Geometry: final body of the model. Coordinates: model frame, mm. A direction names the side the tool comes from. Round coordinates to 2 decimals unless told otherwise and drop trailing zeros. Write each loop counter-clockwise with the first axis right and the second up, starting at its lowest first coordinate (ties: lowest second). Pieces come first, ordered by that corner, then holes.
from build123d import *

# Parameters (mm, degrees)
F0_W          = 70
F0_H          = 60
F1_DEPTH      = 5
F2_R          = 4
F3_DEPTH      = 3
F4_R          = 1.5
F5_DEPTH      = 3.001
F5_DEPTH_BACK = 5
F6_DEPTH      = 3
F7_DEPTH      = 3
F9_DEPTH      = 5
F11_DEPTH     = 3
F13_DEPTH     = 2.5


with BuildPart() as f1:
    # F0 (on Top) → F1 (new body)
    with BuildSketch(Plane.XY):
        Rectangle(F0_W, F0_H)
    extrude(amount=F1_DEPTH)

    # F2 (on face) → F3 (join)
    with BuildSketch(Plane.XY.offset(5)):
        with Locations((-23.7, 23.1)):
            Circle(F2_R)
        with Locations((-25, -25.1)):
            Circle(F2_R)
        with Locations((27.1, 7.9)):
            Circle(F2_R)
        with Locations((27.1, -20)):
            Circle(F2_R)
    extrude(amount=F3_DEPTH)

    # F4 (on face) → F5 (cut, two sides)
    with BuildSketch(Plane.XY.offset(5)) as f5_sk:
        with Locations((-23.7, 23.1)):
            Circle(F4_R)
        with Locations((27.1, 7.9)):
            Circle(F4_R)
        with Locations((27.1, -20)):
            Circle(F4_R)
        with Locations((-25, -25.1)):
            Circle(F4_R)
    extrude(amount=F5_DEPTH, mode=Mode.SUBTRACT)
    extrude(f5_sk.sketch, amount=-F5_DEPTH_BACK, mode=Mode.SUBTRACT)

    # F6 (add): a face of the model
    f6_faces = [f1.faces().sort_by_distance(p)[0] for p in [
        (0, -30, 2.5),
    ]]
    extrude(f6_faces, amount=F6_DEPTH)

    # F7 (add): a face of the model
    f7_faces = [f1.faces().sort_by_distance(p)[0] for p in [
        (0, 30, 2.5),
    ]]
    extrude(f7_faces, amount=F7_DEPTH)

    # F8 (on face) → F9 (cut)
    with BuildSketch(Plane.XY.offset(5)):
        with BuildLine():
            Line((-14.3054683646, -1.7219720702), (-14.0948043176, -1.5533969252))
            ThreePointArc((-14.0948043176, -1.5533969252), (-14.2033899748, -1.6336185148), (-14.3054683646, -1.7219720702))
        make_face()
        with BuildLine():
            Line((0.0942490372, 9.8008030979), (-14.0948043176, -1.5533969252))
            Line((-14.0948043176, -1.5533969252), (-14.3054683646, -1.7219720702))
            ThreePointArc((-14.3054683646, -1.7219720702), (-14.4654537532, -4.1069079107), (-12.0966540364, -4.4267550448))
            Line((-12.0966540364, -4.4267550448), (-11.9406668878, -4.3019831308))
            Line((-11.9406668878, -4.3019831308), (2.8915675597, 7.5621114407))
            Line((2.8915675597, 7.5621114407), (17.79653445, -4.3663210058))
            ThreePointArc((17.79653445, -4.3663210058), (20.2569293491, -4.0927049714), (19.9819440544, -1.632462731))
            Line((19.9819440544, -1.632462731), (5.6767092201, 9.7899068663))
            Line((5.6767092201, 9.7899068663), (19.9831212168, 21.2334034958))
            ThreePointArc((19.9831212168, 21.2334034958), (20.2564890013, 23.6932556011), (17.7966100252, 23.9663814852))
            Line((17.7966100252, 23.9663814852), (2.875636553, 12.0264928184))
            Line((2.875636553, 12.0264928184), (-11.7579023913, 23.711004976))
            ThreePointArc((-11.7579023913, 23.711004976), (-14.2972510493, 23.8856651764), (-14.3249394698, 21.3404675134))
            Line((-14.3249394698, 21.3404675134), (-14.0726513096, 21.1385615113))
            Line((-14.0726513096, 21.1385615113), (0.0942490372, 9.8008030979))
        make_face()
        with BuildLine():
            Line((-11.9406668878, -4.3019831308), (-12.0966540364, -4.4267550448))
            ThreePointArc((-12.0966540364, -4.4267550448), (-12.0168787832, -4.3665965042), (-11.9406668878, -4.3019831308))
        make_face()
        with BuildLine():
            ThreePointArc((-14.3249394698, 21.3404675134), (-14.20346555, 21.2336789942), (-14.0726513096, 21.1385615113))
            Line((-14.0726513096, 21.1385615113), (-14.3249394698, 21.3404675134))
        make_face()
    extrude(amount=-F9_DEPTH, mode=Mode.SUBTRACT)

    # F10 (on face) → F11 (cut)
    with BuildSketch(Plane.XY.offset(5)):
        with BuildLine():
            Line((-1.8575315971, 9.7664474073), (-14.7756829148, -0.5049047258))
            ThreePointArc((-14.7756829148, -0.5049047258), (-15.6013647029, -4.6712575855), (-11.433176099, -5.4876216764))
            Line((-11.433176099, -5.4876216764), (-11.0521931213, -5.1829866811))
            Line((-11.0521931213, -5.1829866811), (2.8911088828, 5.9661144314))
            Line((2.8911088828, 5.9661144314), (16.9025515531, -5.2472313346))
            Line((16.9025515531, -5.2472313346), (17.1329612476, -5.431628019))
            ThreePointArc((17.1329612476, -5.431628019), (21.2784372428, -4.8153147212), (20.7625294306, -0.6561498487))
            Line((20.7625294306, -0.6561498487), (7.6801953311, 9.7954806055))
            Line((7.6801953311, 9.7954806055), (20.7635173832, 20.2569394769))
            ThreePointArc((20.7635173832, 20.2569394769), (21.4878080636, 24.1004643496), (17.7966100252, 25.3936532288))
            Line((17.7966100252, 25.3936532288), (16.4145835398, 24.2947900603))
            Line((16.4145835398, 24.2947900603), (2.9409192439, 13.5817439671))
            Line((2.9409192439, 13.5817439671), (-10.9395035381, 24.6709768489))
            ThreePointArc((-10.9395035381, 24.6709768489), (-15.232323279, 24.7203169337), (-15.1789230669, 20.4275457788))
            Line((-15.1789230669, 20.4275457788), (-14.7762238118, 20.1052659041))
            Line((-14.7762238118, 20.1052659041), (-1.8575315971, 9.7664474073))
        make_face()
        with BuildLine():
            Line((-11.0521931213, -5.1829866811), (-11.433176099, -5.4876216764))
            ThreePointArc((-11.433176099, -5.4876216764), (-11.2364826168, -5.3430605231), (-11.0521931213, -5.1829866811))
        make_face()
        with BuildLine():
            ThreePointArc((-15.1789230669, 20.4275457788), (-14.9845123714, 20.2577354186), (-14.7762238118, 20.1052659041))
            Line((-14.7762238118, 20.1052659041), (-15.1789230669, 20.4275457788))
        make_face()
        with BuildLine():
            Line((17.1329612476, -5.431628019), (16.9025515531, -5.2472313346))
            ThreePointArc((16.9025515531, -5.2472313346), (17.0154876286, -5.3422645814), (17.1329612476, -5.431628019))
        make_face()
        with BuildLine():
            ThreePointArc((17.7966100252, 25.3936532288), (17.0229247716, 24.9481972003), (16.4145835398, 24.2947900603))
            Line((16.4145835398, 24.2947900603), (17.7966100252, 25.3936532288))
        make_face()
    extrude(amount=-F11_DEPTH, mode=Mode.SUBTRACT)

    # F12 (on face) → F13 (cut)
    with BuildSketch(Plane(origin=(0, 0, 0), x_dir=(1, 0, 0), z_dir=(0, 0, -1))):
        Polygon((-24.6492034201, 28.2559903506), (-27.5577695278, 26.981793925), (-27.9085661076, 23.8258035744), (-25.3507965799, 21.9440096494), (-22.4422304722, 23.218206075), (-22.0914338924, 26.3741964256), align=None)
        Polygon((27.1832127793, 23.1743359883), (24.3925507836, 21.659232375), (24.3093380043, 18.4848963867), (27.0167872207, 16.8256640117), (29.8074492164, 18.340767625), (29.8906619957, 21.5151036133), align=None)
        Polygon((27.1178128759, -4.7246234814), (24.3589497063, -6.2968853377), (24.3411368304, -9.4722618563), (27.0821871241, -11.0753765186), (29.8410502937, -9.5031146623), (29.8588631696, -6.3277381437), align=None)
        Polygon((-23.1561984645, -19.9714838624), (-26.1374736836, -21.0647959868), (-26.6812752191, -24.1933121244), (-24.2438015355, -26.2285161376), (-21.2625263164, -25.1352040132), (-20.7187247809, -22.0066878756), align=None)
    extrude(amount=-F13_DEPTH, mode=Mode.SUBTRACT)


solid = f1.part
1) Draft query along Y for faces 4 (the cylindrical face through (20.28, 23.66, 1.01)), 5 (the flat face through (27, 6, 8)), 6 (the flat face through (-27.73, -25.43, 1.23)). Return one class per face: pulls with the +Y half, pulls with the -Y half, needs draft (parallel to the pull), parting line crosses it, or undercut.
2) Section A-A on z = 6.5. Output: boundary loops of the cut face in (x, y), plus the area to 3 significant figures.
3) Section D-D on y = -25.1. Output: boundary loops of the cut face in (x, z), plus the area to 3 significant figures.
4) First-contact query: P1, Ø6, axis at x = -11, y = -5, coming from the +Z side; P2, Ø6, axis at x = -25, y = -16.5, coming from the -Z side; P3, Ø3, axis at x = 28, y = -20, coming from the -Z side; P4, Ø2, axis at x = 27, z = 6.5, coming from the +Y side. Flat tips, straight axial feed; report the tip coordinate or a pass-through.
5) Reachability of faces 1 (the flat face through (0, 0, 5)), 2 (the flat face through (12.93, 4, 1.01)), 3 (the flat face through (-24, -27, 2.5)) from +Z, -Z, +X, -X, +Y, -Y: full face, straight path, thin tool, end or side. Return the list, or none.
6) Section B-B on x = 11.5. Output: boundary loops of the cut face in (y, z).
7) Section C-C on y = -2.5. Output: boundary loops of the cut face in (x, z).
8) Line query: probe 1 along Y at (x, z) = (13.5, 0.5); probe 2 along X at (y, z) = (-0.5, 4.25); probe 3 along X at (y, z) = (-20, 4.55). Output: solid intervals per line, ascending.
Filled in:
1. face 4: undercut
1. face 5: needs draft
1. face 6: undercut
2. outline: circle Ø8 at (-25, -25.1); circle Ø8 at (-23.7, 23.1); circle Ø8 at (27.1, -20); circle Ø8 at (27.1, 7.9); hole circle Ø3 at (-25, -25.1); hole circle Ø3 at (-23.7, 23.1); hole circle Ø3 at (27.1, -20); hole circle Ø3 at (27.1, 7.9)
2. area: 173 mm2
3. outline: (-35, 0) - (-27.77, 0) - (-27.77, 2.5) - (-26.5, 2.5) - (-26.5, 8) - (-29, 8) - (-29, 5) - (-35, 5) - close; (-23.5, 2.5) - (-22.23, 2.5) - (-22.23, 0) - (35, 0) - (35, 5) - (-21, 5) - (-21, 8) - (-23.5, 8) - close
3. area: 344 mm2
4. P1: stops at z = 5
4. P2: stops at z = 0
4. P3: stops at z = 2.5
4. P4: stops at y = 11.9
5. face 1: +Z
5. face 2: +Z, -Z
5. face 3: -Z
6. outline: (-33, 0) - (0.67, 0) - (0.67, 2) - (-0.92, 2) - (-0.92, 5) - (-33, 5) - close; (5.14, 0) - (14.45, 0) - (14.45, 2) - (12.85, 2) - (12.85, 5) - (6.74, 5) - (6.74, 2) - (5.14, 2) - close; (18.93, 0) - (33, 0) - (33, 5) - (20.39, 5) - (20.39, 2) - (18.93, 2) - close
7. outline: (-35, 0) - (-14.79, 0) - (-14.79, 2) - (-16.07, 2) - (-16.07, 5) - (-35, 5) - close; (-9.69, 0) - (15.46, 0) - (15.46, 2) - (13.47, 2) - (13.47, 5) - (-7.7, 5) - (-7.7, 2) - (-9.69, 2) - close; (20.57, 0) - (35, 0) - (35, 5) - (21.85, 5) - (21.85, 2) - (20.57, 2) - close
8. probe 1: y = -33 to -0.93, 3.54 to 16.05, 20.53 to 33
8. probe 2: x = -35 to -14.77, -5.2 to 10.97, 20.57 to 35
8. probe 3: x = -35 to 25.6, 28.6 to 35
